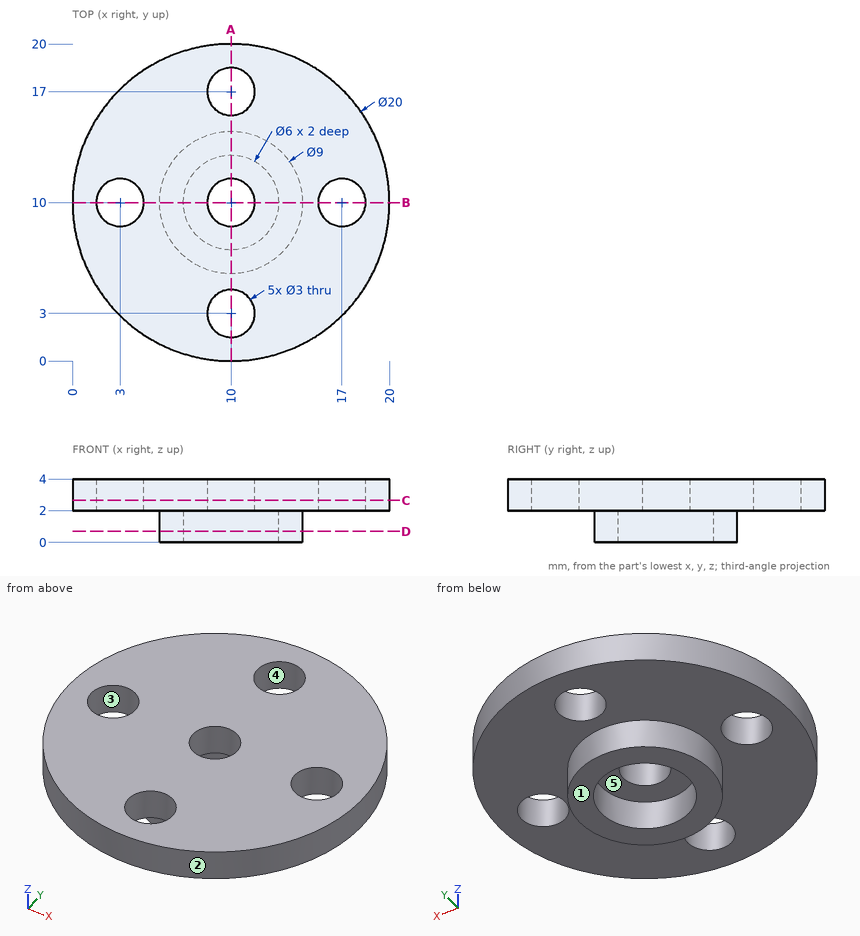
Print and shaded views of the part. All mm, measured from the part's lowest x, y and z. A direction names the side the tool comes from. Coordinates: 2 decimals unless noted, no trailing zeros. Order: outer loops, then holes, each group sorted by start corner. A loop starts at its lowest first (then second) coordinate and runs counter-clockwise, first axis right, second up.
(1) Slice it at A-A, the plane x = 10. Write the cut outline in (y, z), and give its area (3 significant figures).
Check sheet entries:
outline: (0, 2) - (1.5, 2) - (1.5, 4) - (0, 4) - close; (4.5, 2) - (5.5, 2) - (5.5, 0) - (7, 0) - (7, 2) - (8.5, 2) - (8.5, 4) - (4.5, 4) - close; (11.5, 2) - (13, 2) - (13, 0) - (14.5, 0) - (14.5, 2) - (15.5, 2) - (15.5, 4) - (11.5, 4) - close; (18.5, 2) - (20, 2) - (20, 4) - (18.5, 4) - close
area: 28.0 mm2
(2) Pin check, flat tips, straight feed: pin 1 Ø6.5 at (x, y) = (9, 11) entering from -Z; pin 2 Ø3.5 at (x, y) = (10, 10) entering from -Z; pin 3 Ø2.5 at (x, y) = (10, 17) entering from +Z; pin 4 Ø1.5 at (y, z) = (8, 1) entering from +X. Stop position of each tip, or through.
Check sheet entries:
pin 1: stops at z = 0
pin 2: stops at z = 2
pin 3: passes through
pin 4: stops at x = 14.32
(3) Slice it at D-D, the plane z = 0.7. Write the cut outline in (x, y), and give its area (3 significant figures).
Check sheet entries:
outline: circle Ø9 at (10, 10); hole circle Ø6 at (10, 10)
area: 35.3 mm2
(4) Pull direction X, two halves, no side cores. Call the marked faces 1, 2 and 3: pulls with the +X half, pulls with the -X half, needs draft (parallel to the pull), parting line crosses it, or undercut.
Check sheet entries:
face 1: needs draft
face 2: parting line crosses it
face 3: undercut
(5) Tool access for the marked faces 4 and 5: list every direction of +Z, -Z, +X, -X, +Y, -Y with a clear straight run to the whole face (end or side of a thin tool).
Check sheet entries:
face 4: +Z, -Z
face 5: -Z
(6) Probe L1, parallel to Y at x = 10, z = 2.45; L2, parallel to Z at x = 13.25, y = 5.75; L3, parallel to Y at x = 10, z = 0.45. List the from-to ranges inside material, lowest first.
Check sheet entries:
L1: y = 0 to 1.5, 4.5 to 8.5, 11.5 to 15.5, 18.5 to 20
L2: z = 2 to 4
L3: y = 5.5 to 7, 13 to 14.5
(7) Slice it at C-C, the plane z = 2.65. Write the cut outline in (x, y), and give its area (3 significant figures).
Check sheet entries:
outline: circle Ø20 at (10, 10); hole circle Ø3 at (3, 10); hole circle Ø3 at (10, 3); hole circle Ø3 at (10, 10); hole circle Ø3 at (10, 17); hole circle Ø3 at (17, 10)
area: 279 mm2
